Verification items for the finished model (mm, model axes). Round coordinates to 2 decimals unless told otherwise and drop trailing zeros. Write each loop counter-clockwise with the first axis right and the second up, starting at its lowest first coordinate (ties: lowest second). Pieces come first, ordered by that corner, then holes. Notation, with made-up numbers: (57, 6) - (66, 6) arc R15 cw to (66, 29) - close; hole circle Ø7 at (-11.5, 56.5). An arc over 180 degrees is marked (long way). Write each question's results on one line, items separated by ' | '.
```python
from build123d import *

# Parameters (mm, degrees)
SKETCH1_R           = 2.15
SKETCH1_R_2         = 5
BOSS_EXTRUDE1_DEPTH = 1.5875


with BuildPart() as part:
    # Sketch1 → Boss-Extrude1 (new body, symmetric)
    with BuildSketch(Plane(origin=(0, 0, 0), x_dir=(1, 0, 0), z_dir=(0, 1, 0))):
        Polygon((-20, 19.05), (-20, -19.05), (81.6, -19.05), (81.6, -15.875), (107, -15.875), (107, -19.05), (132.4, -19.05), (132.4, -15.875), (157.8, -15.875), (157.8, -19.05), (183.2, -19.05), (183.2, -15.875), (208.6, -15.875), (208.6, -19.05), (234, -19.05), (234, -15.875), (259.4, -15.875), (259.4, -19.05), (310.2, -19.05), (310.2, 19.05), (259.4, 19.05), (259.4, 15.875), (234, 15.875), (234, 19.05), (208.6, 19.05), (208.6, 15.875), (183.2, 15.875), (183.2, 19.05), (157.8, 19.05), (157.8, 15.875), (132.4, 15.875), (132.4, 19.05), (107, 19.05), (107, 15.875), (81.6, 15.875), (81.6, 19.05), align=None)
        with Locations((-8, -8)):
            Circle(SKETCH1_R, mode=Mode.SUBTRACT)
        with Locations((8, -8)):
            Circle(SKETCH1_R, mode=Mode.SUBTRACT)
        with Locations((282.2, -8)):
            Circle(SKETCH1_R, mode=Mode.SUBTRACT)
        with Locations((298.2, -8)):
            Circle(SKETCH1_R, mode=Mode.SUBTRACT)
        Circle(SKETCH1_R_2, mode=Mode.SUBTRACT)
        with Locations((-8, 8)):
            Circle(SKETCH1_R, mode=Mode.SUBTRACT)
        with Locations((8, 8)):
            Circle(SKETCH1_R, mode=Mode.SUBTRACT)
        with Locations((290.2, 0)):
            Circle(SKETCH1_R, mode=Mode.SUBTRACT)
        with Locations((282.2, 8)):
            Circle(SKETCH1_R, mode=Mode.SUBTRACT)
        with Locations((298.2, 8)):
            Circle(SKETCH1_R, mode=Mode.SUBTRACT)
    extrude(amount=BOSS_EXTRUDE1_DEPTH, both=True)


solid = part.part
```
(1) Mould release check, pull along X, two halves, no side actions. Record for faces 1 (the flat face through (143, -1.588, 0)), 2 (the cylindrical face through (-1.08, -0.02, 4.88)): released by +X, released by -X, zero draft, split by the parting line, or undercut.
Answer:
face 1: zero draft | face 2: undercut
(2) Section check A-A (x = 0). Record the cut outline in (y, z), plus the area to 3 significant figures.
Answer:
outline: (-1.59, -19.05) - (1.59, -19.05) - (1.59, -5) - (-1.59, -5) - close; (-1.59, 5) - (1.59, 5) - (1.59, 19.05) - (-1.59, 19.05) - close | area: 89.2 mm2
(3) Section check B-B (y = 0.85). State how many separate pieces and enclosed holes the cut face has, plus the area to 3 significant figures.
Answer:
separate pieces: 1 | enclosed holes: 10 | area: 11,700 mm2
(4) Go/stop test with flat-tipped pins: pin 1 Ø2.5 at (x, z) = (-8, 8) entering from -Y; pin 2 Ø1.6 at (x, y) = (198.5, -0.5) entering from +Z (3 decimals). Record where each tip stops, or that it passes through.
Answer:
pin 1: through | pin 2: z = 15.875
(5) Thickness scan on L1, parallel to X at y = 0.6, z = 8; L2, parallel to X at y = -1.35, z = 17; L3, parallel to X at y = 1.4, z = 0.5. Record the ranges inside material, lowest first.
Answer:
L1: -20 to -10.15, -5.85 to 5.85, 10.15 to 280.05, 284.35 to 296.05, 300.35 to 310.2 | L2: -20 to 81.6, 107 to 132.4, 157.8 to 183.2, 208.6 to 234, 259.4 to 310.2 | L3: -20 to -4.97, 4.97 to 288.11, 292.29 to 310.2
